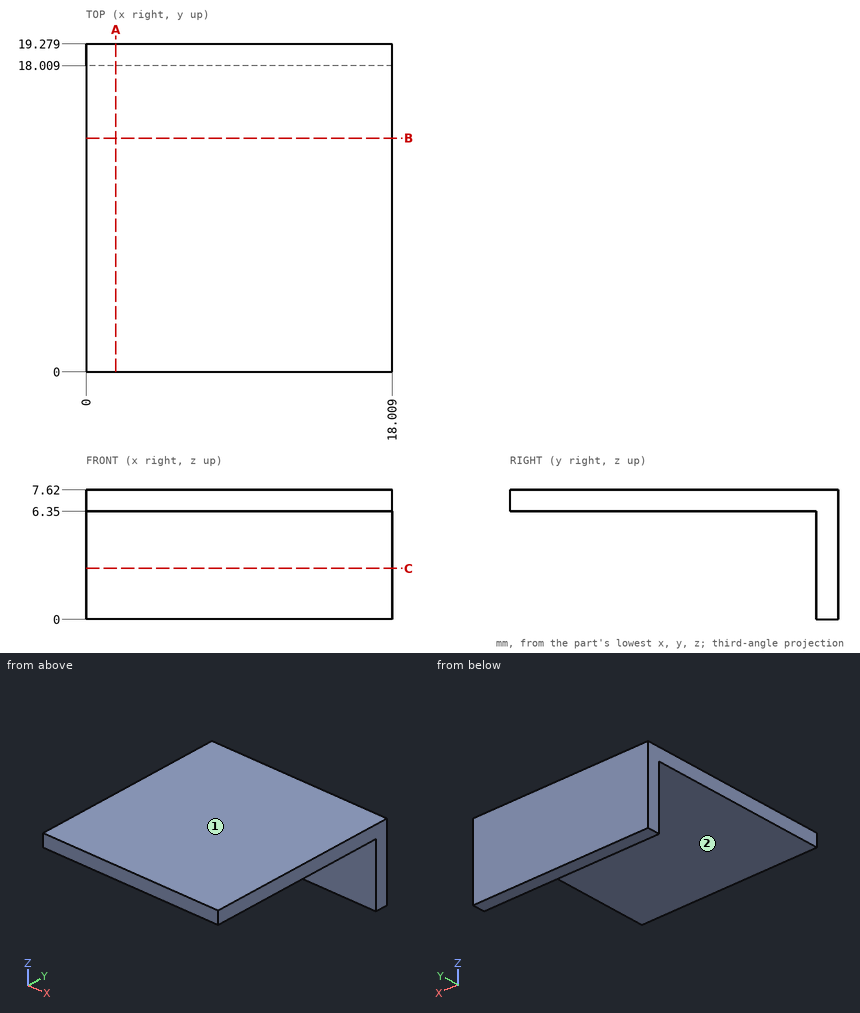
Print and shaded views of the part. All mm, measured from the part's lowest x, y and z. A direction names the side the tool comes from. Round coordinates to 2 decimals unless told otherwise and drop trailing zeros. Write each loop counter-clockwise with the first axis right and the second up, starting at its lowest first coordinate (ties: lowest second). Pieces come first, ordered by that corner, then holes. Notation, with made-up numbers: (-24.75, 19.25) -> (4.25, 19.25) arc R34 ccw to (4.25, 56.25) -> close; hole circle Ø3 at (27.25, 19). An arc over 180 degrees is marked (long way). Return JSON: item names as keys, results as strings. Group by question number.
Q1. Saw through at C-C on z = 3. Write the cut outline in (x, y).
Q2. Pin check, flat tips, straight feed: pin 1 (3 mm diameter, centred on x = 9, z = 4.5, fed in from -Y); pin 2 (1.5 mm diameter, centred on x = 15.5, y = 13.5, fed in from -Z). Stop position of each tip, or through.
Q3. Probe L1, parallel to Z at x = 1, y = 13.25; L2, parallel to Y at x = 11, z = 4.5. List the from-to ranges inside material, lowest first. Write a range as [from, to].
Q4. Which spindle directions (+Z, -Z, +X, -X, +Y, -Y) get a long thin tool onto all of the face, cutting with end or side? Do the marked faces 1 and 2. Say none if no direction does.
Q5. Saw through at B-B on y = 13.75. Write the cut outline in (x, z).
Q6. Saw through at A-A on x = 1.75. Write the cut outline in (y, z).
Answer:
{
 "1": {"outline": "(0, 18.01) -> (18.01, 18.01) -> (18.01, 19.28) -> (0, 19.28) -> close"},
 "2": {"pin 1": "y = 18.01", "pin 2": "z = 6.35"},
 "3": {"L1": "[6.35, 7.62]", "L2": "[18.01, 19.28]"},
 "4": {"face 1": "+Z, +X, -X, +Y, -Y", "face 2": "-Z, +X, -X, -Y"},
 "5": {"outline": "(0, 6.35) -> (18.01, 6.35) -> (18.01, 7.62) -> (0, 7.62) -> close"},
 "6": {"outline": "(0, 6.35) -> (18.01, 6.35) -> (18.01, 0) -> (19.28, 0) -> (19.28, 7.62) -> (0, 7.62) -> close"}
}
